```python
from build123d import *

# Parameters (mm, degrees)
SKETCH1_R               = 21.5
BOSS_EXTRUDE1_DEPTH     = 4
SKETCH2_R               = 21.5
SKETCH2_R_2             = 12.625
BOSS_EXTRUDE2_DEPTH     = 1
SKETCH3_R               = 3.429
CUT_EXTRUDE1_DEPTH      = 31.813957876
CUT_EXTRUDE1_DEPTH_BACK = 31.813957876
SKETCH4_R               = 3.429
BOSS_EXTRUDE3_DEPTH     = 34
CHAMFER1_SIZE           = 0.5


with BuildPart() as part:
    # Sketch1 → Boss-Extrude1 (new body)
    with BuildSketch(Plane(origin=(0, 0, 0), x_dir=(0, 0, -1), z_dir=(1, 0, 0))):
        Circle(SKETCH1_R)
    extrude(amount=BOSS_EXTRUDE1_DEPTH)

    # Sketch2 → Boss-Extrude2 (add)
    with BuildSketch(Plane(origin=(4, 0, 0), x_dir=(0, 0, -1), z_dir=(1, 0, 0))):
        Circle(SKETCH2_R)
        Circle(SKETCH2_R_2, mode=Mode.SUBTRACT)
    extrude(amount=BOSS_EXTRUDE2_DEPTH)

    # Sketch3 → Cut-Extrude1 (cut, two sides)
    with BuildSketch(Plane.ZY) as cut_extrude1_sk:
        with Locations(Location((0, 0, 0), (0, 0, 180))):
            Circle(SKETCH3_R)
    extrude(amount=CUT_EXTRUDE1_DEPTH, mode=Mode.SUBTRACT)
    extrude(cut_extrude1_sk.sketch, amount=-CUT_EXTRUDE1_DEPTH_BACK, mode=Mode.SUBTRACT)

    # Sketch4 → Boss-Extrude3 (add)
    with BuildSketch(Plane(origin=(4, 0, 0), x_dir=(0, 0, -1), z_dir=(1, 0, 0))):
        Polygon((4.965212315, -8.6), (9.93042463, 0), (4.965212315, 8.6), (-4.965212315, 8.6), (-9.93042463, 0), (-4.965212315, -8.6), align=None)
        Circle(SKETCH4_R, mode=Mode.SUBTRACT)
    extrude(amount=BOSS_EXTRUDE3_DEPTH)

    # Chamfer1
    chamfer1_edges = [part.edges().sort_by_distance(p)[0] for p in [
        (5, 0, 21.5),
    ]]
    chamfer(chamfer1_edges, length=CHAMFER1_SIZE)


solid = part.part
```
Can you work these out from the model? Positions are in its coordinate system, mm. A direction names the side the tool comes from. Coordinates: 2 decimals unless noted, no trailing zeros. Order: outer loops, then holes, each group sorted by start corner. A loop starts at its lowest first (then second) coordinate and runs counter-clockwise, first axis right, second up.
1. I'm going to push flat-ended pins straight in: pin 1 (8 mm diameter, centred on x = 19, y = -4.5, fed in from +Z); pin 2 (12 mm diameter, centred on x = 27.5, y = -2.5, fed in from +Z); pin 3 (11 mm diameter, centred on x = 18, z = 2, fed in from +Y). Where does each tip first touch, or does it pass through?
2. I need wall thicknesses on line 1 (Y direction, x = 4.5, z = 0) (3 decimals); line 2 (Y direction, x = 9, z = 0); line 3 (X direction, y = 15, z = 2). Which ranges of each line are inside material? Lowest first, please.
3. If we section it at A-A (x = 14): Please give me the cut outline in (y, z), then the cut area to 3 significant figures.
4. Thinking about a two-plate mould opening in Z: for faces 1 (the face through (18.73, -3.35, 0.74)), 2 (the face through (5, -9.04, -9.04)), 3 (the face through (4, -3, 9)), 4 (the face through (2.218, 21.317, 2.799)), which applies, +Z half, -Z half, draft (parallel to the pull), parting line (faces both ways), or undercut?
5. If we section it at B-B (z = 0): Please give me the cut outline in (x, y) (3 decimals).
6. For faces 5 (the face through (0, 0, -4)), 6 (the face through (4.493, -12.325, 2.737)), which set-ups out of +Z, -Z, +X, -X, +Y, -Y let a thin tool reach every point of the face, with its end or its side?
Entries:
1. pin 1: stops at z = 9.64
1. pin 2: stops at z = 9.93
1. pin 3: stops at y = 8.6
2. line 1: y = -21.5 to -12.625, -8.6 to -3.429, 3.429 to 8.6, 12.625 to 21.5
2. line 2: y = -8.6 to -3.43, 3.43 to 8.6
2. line 3: x = 0 to 5
3. outline: (-8.6, -4.97) - (0, -9.93) - (8.6, -4.97) - (8.6, 4.97) - (0, 9.93) - (-8.6, 4.97) - close; hole circle Ø6.86 at (0, 0)
3. area: 219 mm2
4. face 1: undercut
4. face 2: draft
4. face 3: undercut
4. face 4: parting line
5. outline: (0, -21.5) - (4.5, -21.5) - (5, -21) - (5, -12.625) - (4, -12.625) - (4, -8.6) - (38, -8.6) - (38, -3.429) - (0, -3.429) - close; (0, 3.429) - (38, 3.429) - (38, 8.6) - (4, 8.6) - (4, 12.625) - (5, 12.625) - (5, 21) - (4.5, 21.5) - (0, 21.5) - close
6. face 5: +Z, -Z, -X, +Y, -Y
6. face 6: +X
